```python
from build123d import *

# Parameters (mm, degrees)
F2_DEPTH  = 2.5
F4_DEPTH  = 2.5
F8_W      = 5
F8_H      = 3.25
F9_DEPTH  = 2
F10_W     = 5
F10_H     = 7.5
F11_DEPTH = 2


with BuildPart() as f2:
    # F1 (on Right) → F2 (new body)
    with BuildSketch(Plane.YZ):
        with BuildLine():
            ThreePointArc((7.5, -6), (1.5, 0), (7.5, 6))
            Line((7.5, 6), (-7.5, 6))
            ThreePointArc((-7.5, 6), (-13.5, 0), (-7.5, -6))
            Line((-7.5, -6), (7.5, -6))
        make_face()
    extrude(amount=-F2_DEPTH)

    # F0 (on Right) → F4 (join)
    with BuildSketch(Plane.YZ):
        Polygon((0, 6), (0, -6), (15, -6), (15, 1), (10, 6), align=None)
    extrude(amount=F4_DEPTH)

    # F6 (on offset) → F7 (revolve, cut)
    with BuildSketch(Plane.XZ.offset(-9.77)):
        with BuildLine():
            Line((-2.5325156748, 2.5), (-2.5325156748, 0))
            Line((-2.5325156748, 0), (1.556239127, 0))
            ThreePointArc((1.556239127, 0), (1.1353956611, 1.4724028169), (0, 2.5))
            Line((0, 2.5), (-2.5325156748, 2.5))
        make_face()
    revolve(axis=Axis((-10.801910348, 9.77, 0), (1, 0, 0)), mode=Mode.SUBTRACT)

    # F8 (on face) → F9 (join)
    with BuildSketch(Plane.XY.offset(6)):
        with Locations((-5, 3.75)):
            Rectangle(F8_W, F8_H)
    extrude(amount=-F9_DEPTH)

    # F10 (on face) → F11 (join)
    with BuildSketch(Plane(origin=(0, 0, -6), x_dir=(1, 0, 0), z_dir=(0, 0, -1))):
        with Locations((-5, -3.75)):
            Rectangle(F10_W, F10_H)
    extrude(amount=-F11_DEPTH)

    # F14 (on offset) → F15 (revolve)
    with BuildSketch(Plane.XZ.offset(7.5)):
        with BuildLine():
            Line((0, 0), (1.524425623, 0))
            ThreePointArc((1.524425623, 0), (1.1132612082, 1.4640588684), (0, 2.5))
            Line((0, 2.5), (0, 0))
        make_face()
    revolve(axis=Axis((-0.2374296736, -7.5, 0), (1, 0, 0)))

    # F16: F2 across plane


with BuildPart() as f2_1:
    add(f2.part)
    add(f2.part.mirror(Plane(origin=(-7.5, 3.75, -5), x_dir=(0, -1, 0), z_dir=(-1, 0, 0))))


solid = f2_1.part
```
Here's how the part is built. I have some questions about the finished solid (model axes, mm). A direction names the side the tool comes from. Give positions to 0.01 mm unless a question says otherwise; leave off trailing zeros. Write each loop counter-clockwise with the first axis right and the second up, starting at its lowest first coordinate (ties: lowest second). Pieces come first, ordered by that corner, then holes. Notation, with made-up numbers: (1, 32.25) -> (34, 32.25) arc R16 cw to (34, 61.25) -> close; hole circle Ø8 at (48.25, 25.5). An arc over 180 degrees is marked (long way). Write each question's results on one line, items separated by ' | '.
Item 1: Suppose I cut it at A-A on x = 0.75. Write out the boundary of the cut face in (y, z).
Output:
outline: circle Ø3.88 at (-7.5, 0); (0, -6) -> (15, -6) -> (15, 1) -> (10, 6) -> (0, 6) -> close; hole circle Ø3.92 at (9.77, 0)
Item 2: Suppose I cut it at D-D on x = -3. Write out the boundary of the cut face in (y, z) (3 decimals), plus the area to 3 significant figures.
Output:
outline: (0, -6) -> (7.5, -6) -> (7.5, -4) -> (0, -4) -> close; (2.125, 4) -> (5.375, 4) -> (5.375, 6) -> (2.125, 6) -> close | area: 21.5 mm^2
Item 3: Suppose I cut it at C-C on y = -4.5. Write out the boundary of the cut face in (x, z).
Output:
outline: (-15, -6) -> (-12.5, -6) -> (-12.5, 6) -> (-15, 6) -> close; (-2.5, -6) -> (0, -6) -> (0, 6) -> (-2.5, 6) -> close
Item 4: Suppose I cut it at B-B on z = 0. Write out the boundary of the cut face in (x, y).
Output:
outline: (-17.5, 0) -> (-15, 0) -> (-15, -5) arc R2.81 ccw to (-15, -10) -> (-15, -13.5) -> (-12.5, -13.5) -> (-12.5, 1.5) -> (-15, 1.5) -> (-15, 7.27) arc R2.79 cw to (-15, 12.27) -> (-15, 15) -> (-17.5, 15) -> close; (-2.5, -13.5) -> (0, -13.5) -> (0, -10) arc R2.81 ccw to (0, -5) -> (0, 0) -> (2.5, 0) -> (2.5, 15) -> (0, 15) -> (0, 12.27) arc R2.79 cw to (0, 7.27) -> (0, 1.5) -> (-2.5, 1.5) -> close
Item 5: We'd pull the mould along Y, two halves only. Please class faces 1 (the face through (-7, 5.375, 5)), 2 (the face through (-7, 0, -5)), 3 (the face through (2.5, 7, 0)), 4 (the face through (1, 0, 0)): pulls with the +Y half, pulls with the -Y half, needs draft (parallel to the pull), parting line crosses it, or undercut.
Output:
face 1: pulls with the +Y half | face 2: pulls with the -Y half | face 3: needs draft | face 4: undercut
Item 6: If I drill on L1, parallel to X at y = -11.75, z = -0.25; L2, parallel to X at y = 3.5, z = -0.5; L3, parallel to Z at x = -7, y = 2, over which ranges is the centre line in solid material (lowest first)?
Output:
L1: x = -15 to -12.5, -2.5 to 0 | L2: x = -17.5 to -15, 0 to 2.5 | L3: z = -6 to -4
Item 7: For pin 1 Ø6 at (x, z) = (-10, -2) entering from +Y; pin 2 Ø1 at (y, z) = (-1, -3.5) entering from +X; pin 3 Ø3.5 at (y, z) = (-8, 2) entering from +X, each with a flat end and sliding along its axis, tell me the tip position at first contact or that it passes through.
Output:
pin 1: stops at y = 7.5 | pin 2: stops at x = 0 | pin 3: stops at x = 1.51
Item 8: On a 3-axis mill with a long thin cutter (end or side, diameter ignored), from which of +Z, -Z, +X, -X, +Y, -Y can I reach the whole of each face in a straight line? I mean faces 5 (the face through (-16, 13, 3)), 6 (the face through (-2.5, 4.4, 4.6)), 7 (the face through (-7, 7.5, -5)). Say none if no direction works.
Output:
face 5: +Z, +X, -X, +Y | face 6: +Y | face 7: +Z, -Z, +Y
